Source: CAD feature listing. Evaluate the final solid. Frame: model axes, mm. A direction names the side the tool comes from. Coordinates: 2 decimals unless noted, no trailing zeros. Order: outer loops, then holes, each group sorted by start corner. A loop starts at its lowest first (then second) coordinate and runs counter-clockwise, first axis right, second up.
```python
from build123d import *

# Parameters (mm, degrees)
SKETCH1_W           = 17.76
SKETCH1_H           = 5
BOSS_EXTRUDE1_DEPTH = 1.5
SKETCH2_R           = 1.185
BOSS_EXTRUDE2_DEPTH = 2.5
SKETCH3_R           = 2.275
SKETCH3_R_2         = 1.6
SKETCH3_R_3         = 1.601514513
BOSS_EXTRUDE3_DEPTH = 7.76


with BuildPart() as part:
    # Sketch1 → Boss-Extrude1 (new body)
    with BuildSketch(Plane.XY):
        with Locations((8.88, 2.5)):
            Rectangle(SKETCH1_W, SKETCH1_H)
    extrude(amount=BOSS_EXTRUDE1_DEPTH)

    # Sketch2 → Boss-Extrude2 (add)
    with BuildSketch(Plane.XY.offset(1.5)):
        with Locations((2.54, 2.5)):
            Circle(SKETCH2_R)
        with Locations((15.24, 2.5)):
            Circle(SKETCH2_R)
    extrude(amount=BOSS_EXTRUDE2_DEPTH)

    # Sketch3 → Boss-Extrude3 (add)
    # profile 1 of 2: a face of its own
    with BuildSketch(Plane(origin=(0, 0, 0), x_dir=(-1, 0, 0), z_dir=(0, 0, -1))):
        with Locations(Location((-12.875, 2.5, 0), (0, 0, 180))):
            Circle(SKETCH3_R)
        with Locations((-12.875, 2.5)):
            Circle(SKETCH3_R_2, mode=Mode.SUBTRACT)
    # profile 2 of 2: a face of its own
    with BuildSketch(Plane(origin=(0, 0, 0), x_dir=(-1, 0, 0), z_dir=(0, 0, -1))):
        with Locations(Location((-4.91, 2.5, 0), (0, 0, 180))):
            Circle(SKETCH3_R)
        with Locations((-4.91, 2.5)):
            Circle(SKETCH3_R_3, mode=Mode.SUBTRACT)
    extrude(amount=BOSS_EXTRUDE3_DEPTH)


solid = part.part
```
1. Section query B-B, the plane y = 2.5. Output: boundary loops of the cut face in (x, z) (3 decimals), plus the area to 3 significant figures.
2. Section query A-A, the plane z = 3.25. Output: boundary loops of the cut face in (x, y) (3 decimals).
3. Access query for faces 4 (the cylindrical face through (3.635, 2.046, 2.732)), 5 (the flat face through (15, 3, 4)), 6 (the cylindrical face through (6.51, 2.57, -3.83)). Directions: +Z, -Z, +X, -X, +Y, -Y. A direction counts if a zero-diameter tool reaches every point of the face in a straight line with its end or side. Return the directions, or none.
4. Section query C-C, the plane z = -0.75. Output: boundary loops of the cut face in (x, y) (3 decimals).
5. Contact query for flat-ended pins moving along their axis: P1, Ø3, axis at x = 14, y = 0.5, coming from the +Z side; P2, Ø3, axis at y = 3, z = -5, coming from the -X side (3 decimals); P3, Ø6, axis at x = 6, z = -3.5, coming from the +Y side (3 decimals); P4, Ø2.5, axis at x = 6, y = 3, coming from the +Z side. Output: stop coordinate, or through.
6. Material intervals for line 1 along X through (y, z) = (1.15, -6.5); line 2 along Z through (x, y) = (9, 3.4); line 3 along Y through (x, z) = (4.91, -4.5) (3 decimals), sorted ascending.
7. Section query D-D, the plane x = 4.5. Output: boundary loops of the cut face in (y, z).
8. Draft query along X for faces 1 (the flat face through (3, 3, -7.76)), 2 (the flat face through (17.76, 2, 1)), 3 (the flat face through (13, 3, 0)). Return one class per face: +X half, -X half, draft (parallel to the pull), parting line (faces both ways), or undercut.
Answer key:
1. outline: (0, 0) - (2.635, 0) - (2.635, -7.76) - (3.308, -7.76) - (3.308, 0) - (6.512, 0) - (6.512, -7.76) - (7.185, -7.76) - (7.185, 0) - (10.6, 0) - (10.6, -7.76) - (11.275, -7.76) - (11.275, 0) - (14.475, 0) - (14.475, -7.76) - (15.15, -7.76) - (15.15, 0) - (17.76, 0) - (17.76, 1.5) - (16.425, 1.5) - (16.425, 4) - (14.055, 4) - (14.055, 1.5) - (3.725, 1.5) - (3.725, 4) - (1.355, 4) - (1.355, 1.5) - (0, 1.5) - close
1. area: 59.4 mm2
2. outline: circle Ø2.37 at (2.54, 2.5); circle Ø2.37 at (15.24, 2.5)
3. face 4: +Z
3. face 5: +Z, +X, -X, +Y, -Y
3. face 6: -Z
4. outline: circle Ø4.55 at (4.91, 2.5); circle Ø4.55 at (12.875, 2.5); hole circle Ø3.203 at (4.91, 2.5); hole circle Ø3.2 at (12.875, 2.5)
5. P1: stops at z = 4
5. P2: stops at x = 2.635
5. P3: stops at y = 4.775
5. P4: stops at z = 1.5
6. line 1: x = 3.08 to 4.05, 5.77 to 6.74, 11.04 to 12.02, 13.73 to 14.71
6. line 2: z = 0 to 1.5
6. line 3: y = 0.225 to 0.898, 4.102 to 4.775
7. outline: (0, 0) - (0.26, 0) - (0.26, -7.76) - (0.95, -7.76) - (0.95, 0) - (4.05, 0) - (4.05, -7.76) - (4.74, -7.76) - (4.74, 0) - (5, 0) - (5, 1.5) - (0, 1.5) - close
8. face 1: draft
8. face 2: +X half
8. face 3: undercut
